Autodesk Inventor part; units mm, degrees
ref_plane "YZ Plane" through (0, 0, 0) normal (1, 0, 0) x (0, 1, 0)
ref_plane "XZ Plane" through (0, 0, 0) normal (0, 1, 0) x (-1, 0, 0)
ref_plane "XY Plane" through (0, 0, 0) normal (0, 0, 1) x (1, 0, 0)
sketch "Sketch1" plane through (0, 0, 0) normal (0, 0, 1) x (1, 0, 0)
  line L0 (-206.4864, -0.0159) -> (-206.4864, -68.5959) construction
  line L1 (-206.4864, -0.0159) -> (-222.6154, -0.0159) construction
  line L2 (-222.6154, -0.0159) -> (-222.6154, -68.5959) construction
  line L3 (-206.4864, -68.5959) -> (-222.6154, -68.5959) construction
  circle A0 centre (-214.5636, -21.8091) radius 3.3735 construction
  circle A1 centre (-214.5636, -46.8027) radius 3.3735 construction
  circle A2 centre (-214.5636, -9.3123) radius 2.5 construction
  circle A3 centre (-214.5636, -34.3059) radius 2.5 construction
  circle A4 centre (-214.5636, -59.2995) radius 2.5 construction
  line L4 (0.4039, -68.5877) -> (0.4039, -0.0077) construction
  line L5 (0.4039, -68.5877) -> (16.5329, -68.5877) construction
  line L6 (16.5329, -68.5877) -> (16.5329, -0.0077) construction
  line L7 (0.4039, -0.0077) -> (16.5329, -0.0077) construction
  circle A5 centre (8.4811, -46.7945) radius 3.3735 construction
  circle A6 centre (8.4811, -21.8009) radius 3.3735 construction
  circle A7 centre (8.4811, -59.2913) radius 2.5 construction
  circle A8 centre (8.4811, -34.2977) radius 2.5 construction
  circle A9 centre (8.4811, -9.3041) radius 2.5 construction
  line L8 (-223.0413, -0.0159) -> (16.9587, -0.0159)
  line L9 (16.9587, -0.0159) -> (16.9587, -68.5959)
  line L10 (16.9587, -68.5959) -> (-223.0413, -68.5959)
  line L11 (-223.0413, -68.5959) -> (-223.0413, -0.0159)
  line L12 (-103.0413, -534.726) -> (-103.0413, 430.7972) construction
  point P0 (0, 0)
  dimension "d0" = 240
  dimension "d23" = 120
extrude "Extrusion1" add sketch "Sketch1" along normal blind 12
sketch "Sketch3" plane through (0, 0, 0) normal (0, 0, -1) x (-1, 0, 0)
  circle A0 centre (65.542, -46.7868) radius 2.5 construction
  circle A1 centre (65.542, -21.7868) radius 2.5 construction
  circle A2 centre (165.542, -21.7868) radius 2.5 construction
  circle A3 centre (165.542, -46.7868) radius 2.5 construction
  circle A4 centre (140.542, -46.7868) radius 2.5 construction
  circle A5 centre (140.542, -21.7868) radius 2.5 construction
  circle A6 centre (65.542, -46.7868) radius 2.5 construction
  circle A7 centre (65.542, -21.7868) radius 2.5 construction
  circle A8 centre (40.542, -21.7868) radius 2.5 construction
  circle A9 centre (40.542, -46.7868) radius 2.5 construction
  point P0 (0, 0)
sketch "Sketch4" plane through (0, 0, 0) normal (0, 0, -1) x (-1, 0, 0)
  circle A0 centre (65.5413, -59.3059) radius 2.5 construction
  circle A1 centre (40.5413, -59.3059) radius 2.5 construction
  circle A2 centre (140.5413, -9.3059) radius 2.5 construction
  circle A3 centre (115.5413, -9.3059) radius 2.5 construction
  line L0 (40.5413, -59.3059) -> (172.5963, -59.3059) construction
  line L1 (167.5124, -9.3059) -> (3.0086, -9.3059) construction
  line L2 (223.0413, -0.0159) -> (-16.9587, -0.0159) construction
  line L3 (38.0413, -9.3059) -> (168.0413, -9.3059) construction
  line L4 (38.0413, -12.3559) -> (168.0413, -12.3559)
  line L5 (168.0413, -6.2559) -> (38.0413, -6.2559)
  arc A4 (38.0413, -6.2559) -> (38.0413, -12.3559) centre (38.0413, -9.3059) ccw
  arc A5 (168.0413, -12.3559) -> (168.0413, -6.2559) centre (168.0413, -9.3059) ccw
  line L6 (103.0413, 455.7975) -> (103.0413, -509.7257) construction
  line L7 (38.0413, -59.3059) -> (168.0413, -59.3059) construction
  line L8 (38.0413, -62.3559) -> (168.0413, -62.3559)
  line L9 (168.0413, -56.2559) -> (38.0413, -56.2559)
  arc A6 (38.0413, -56.2559) -> (38.0413, -62.3559) centre (38.0413, -59.3059) ccw
  arc A7 (168.0413, -62.3559) -> (168.0413, -56.2559) centre (168.0413, -59.3059) ccw
  point P0 (0, 0)
  point P1 (-16.9587, -0.0159)
  point P2 (103.0413, -9.3059)
  point P3 (103.0413, -59.3059)
  dimension "d10" = 9.29
  dimension "d11" = 6.1
  dimension "d12" = 65
  dimension "d13" = 65
  dimension "d14" = 6.1
  dimension "d15" = 65
  dimension "d16" = 65
extrude "Extrusion2" cut sketch "Sketch4" against normal blind 12
sketch "Sketch5" plane through (0, 0, 0) normal (0, 0, -1) x (-1, 0, 0)
  line L0 (45.6373, -31.0674) -> (77.6413, -31.0674) construction
  arc A0 (168.0413, -12.3559) -> (168.0413, -6.2559) centre (168.0413, -9.3059) ccw construction
  arc A1 (168.0413, -62.3559) -> (168.0413, -56.2559) centre (168.0413, -59.3059) ccw construction
  arc A2 (38.0413, -6.2559) -> (38.0413, -12.3559) centre (38.0413, -9.3059) ccw construction
  arc A3 (38.0413, -56.2559) -> (38.0413, -62.3559) centre (38.0413, -59.3059) ccw construction
  line L1 (38.0413, -9.3059) -> (168.0413, -9.3059) construction
  line L2 (-16.9587, -0.0159) -> (223.0413, -0.0159)
  line L3 (38.0413, -14.5559) -> (168.0413, -14.5559)
  line L4 (168.0413, -4.0559) -> (38.0413, -4.0559)
  arc A4 (38.0413, -4.0559) -> (38.0413, -14.5559) centre (38.0413, -9.3059) ccw
  arc A5 (168.0413, -14.5559) -> (168.0413, -4.0559) centre (168.0413, -9.3059) ccw
  line L5 (38.0413, -59.3059) -> (168.0413, -59.3059) construction
  line L6 (38.0413, -64.5559) -> (168.0413, -64.5559)
  line L7 (168.0413, -54.0559) -> (38.0413, -54.0559)
  arc A6 (38.0413, -54.0559) -> (38.0413, -64.5559) centre (38.0413, -59.3059) ccw
  arc A7 (168.0413, -64.5559) -> (168.0413, -54.0559) centre (168.0413, -59.3059) ccw
  point P0 (0, 0)
  point P1 (103.0413, -9.3059)
  point P2 (103.0413, -59.3059)
  dimension "d19" = 10.5
  dimension "d20" = 10.5
extrude "Extrusion3" cut sketch "Sketch5" against normal blind 6.5
sketch "Sketch6" plane through (0, 0, 12) normal (0, 0, 1) x (1, 0, 0)
  line L0 (0.4039, -68.5877) -> (0.4039, -0.0077) construction
  line L1 (0.4039, -68.5877) -> (16.5329, -68.5877) construction
  line L2 (16.5329, -68.5877) -> (16.5329, -0.0077) construction
  line L3 (0.4039, -0.0077) -> (16.5329, -0.0077) construction
  circle A0 centre (8.4811, -46.7945) radius 3.3735 construction
  circle A1 centre (8.4811, -21.8009) radius 3.3735 construction
  circle A2 centre (8.4811, -59.2913) radius 2.5 construction
  circle A3 centre (8.4811, -34.2977) radius 2.5 construction
  circle A4 centre (8.4811, -9.3041) radius 2.5 construction
  line L4 (-206.4864, -0.0159) -> (-206.4864, -68.5959) construction
  line L5 (-206.4864, -0.0159) -> (-222.6154, -0.0159) construction
  line L6 (-222.6154, -0.0159) -> (-222.6154, -68.5959) construction
  line L7 (-206.4864, -68.5959) -> (-222.6154, -68.5959) construction
  circle A5 centre (-214.5636, -21.8091) radius 3.3735 construction
  circle A6 centre (-214.5636, -46.8027) radius 3.3735 construction
  circle A7 centre (-214.5636, -9.3123) radius 2.5 construction
  circle A8 centre (-214.5636, -34.3059) radius 2.5 construction
  circle A9 centre (-214.5636, -59.2995) radius 2.5 construction
  point P0 (0, 0)
hole "Hole2" at (8.4811, -59.2913, 12) at (8.4811, -34.2977, 12) at (8.4811, -9.3041, 12) at (-214.5636, -59.2995, 12) at (-214.5636, -34.3059, 12) at (-214.5636, -9.3123, 12) direction (0, 0, -1) diameter 6.1 depth 20 tip angle 118 counterbore diameter 11.5 counterbore depth 7
properties part number "ASI_mesoSPIM_Bridge"
Build history of the part. All positions in model axes, mm. A direction names the side the tool comes from. Give positions to 0.01 mm unless a question says otherwise; leave off trailing zeros. Order: outer loops, then holes, each group sorted by start corner. A loop starts at its lowest first (then second) coordinate and runs counter-clockwise, first axis right, second up. Notation, with made-up numbers: M -19,-15 L 10,-15 A8 cw 10,-5 Z; hole C 62,51.25 d5. An arc over 180 degrees is marked long. Return JSON: item names as keys, results as strings.
Q1. Band-saw the part on D-D (z = 2.5). Count the separate pieces of the cut face and the enclosed holes in it, then the cut area to 3 significant figures.
Answer list:
{"separate pieces": "1", "enclosed holes": "8", "area": "13,400 mm^2"}
Q2. Band-saw the part on A-A (x = -84). Give the cut face in (y, z).
Answer list:
{"outline": "M -68.6,0 L -64.56,0 L -64.56,6.5 L -62.36,6.5 L -62.36,12 L -68.6,12 Z; M -56.26,6.5 L -54.06,6.5 L -54.06,0 L -14.56,0 L -14.56,6.5 L -12.36,6.5 L -12.36,12 L -56.26,12 Z; M -6.26,6.5 L -4.06,6.5 L -4.06,0 L -0.02,0 L -0.02,12 L -6.26,12 Z"}
Q3. Flat gauge pins, fed straight in: pin 1 (3.5 mm diameter, centred on x = -215.5, y = -7.5, fed in from +Z); pin 2 (3.5 mm diameter, centred on x = 8.48, y = -34.3, fed in from +Z); pin 3 (13 mm diameter, centred on x = 8.48, y = -34.3, fed in from +Z). Where does each tip first touch, or does it go through?
Answer list:
{"pin 1": "stops at z = 5", "pin 2": "passes through", "pin 3": "stops at z = 12"}
Q4. Wall check: probe 1 along Y at (x, z) = (-165, 7); probe 2 along Y at (x, z) = (-114.5, 2.75); probe 3 along Y at (x, z) = (6, 1.5). Give the ranges that are in metal, low to high. Write a range as from..to.
Answer list:
{"probe 1": "y = -68.6..-62.36, -56.26..-12.36, -6.26..-0.02", "probe 2": "y = -68.6..-64.56, -54.06..-14.56, -4.06..-0.02", "probe 3": "y = -68.6..-61.07, -57.52..-36.07, -32.52..-11.08, -7.53..-0.02"}
Q5. Band-saw the part on B-B (y = -59). Give the cut face in (x, z), then the cut area to 3 significant figures.
Answer list:
{"outline": "M -223.04,0 L -217.6,0 L -217.6,5 L -220.31,5 L -220.31,12 L -223.04,12 Z; M -211.53,0 L -173.28,0 L -173.28,6.5 L -171.08,6.5 L -171.08,12 L -208.82,12 L -208.82,5 L -211.53,5 Z; M -35.01,6.5 L -32.8,6.5 L -32.8,0 L 5.45,0 L 5.45,5 L 2.74,5 L 2.74,12 L -35.01,12 Z; M 11.52,0 L 16.96,0 L 16.96,12 L 14.22,12 L 14.22,5 L 11.52,5 Z", "area": "997 mm^2"}
Q6. Two-plate mould, pull along X, no slides. Class faces 5 (the face through (-102, -14.556, 3)), 6 (the face through (16.959, -34, 6)), 7 (the face through (-105, -34, 12)): pulls with the +X half, pulls with the -X half, needs draft (parallel to the pull), parting line crosses it, or undercut.
Answer list:
{"face 5": "undercut", "face 6": "pulls with the +X half", "face 7": "needs draft"}
Q7. Band-saw the part on C-C (y = -35). Give the cut face in (x, z).
Answer list:
{"outline": "M -223.04,0 L -217.53,0 L -217.53,5 L -220.27,5 L -220.27,12 L -223.04,12 Z; M -211.59,0 L 5.51,0 L 5.51,5 L 2.77,5 L 2.77,12 L -208.86,12 L -208.86,5 L -211.59,5 Z; M 11.45,0 L 16.96,0 L 16.96,12 L 14.19,12 L 14.19,5 L 11.45,5 Z"}
Q8. 3-axis set-ups, long thin cutter, end or side, ignore diameter. For faces 1 (the face through (8.228, -28.553, 8.451)), 2 (the face through (-102, -64.556, 3)), 3 (the face through (-101, -68.596, 6)), 4 (the face through (-171.09, -59.37, 9.21)): which of +Z, -Z, +X, -X, +Y, -Y reach the whole face in a straight line?
Answer list:
{"face 1": "+Z", "face 2": "-Z", "face 3": "+Z, -Z, +X, -X, -Y", "face 4": "+Z, -Z"}
